from build123d import *

# Parameters (mm, degrees)
BOSS_EXTRUDE1_DEPTH     = 28.8
SKETCH3_R               = 3
SKETCH3_R_2             = 1.25
BOSS_EXTRUDE2_DEPTH     = 4
BOSS_EXTRUDE3_DEPTH     = 7.5
SKETCH5_W               = 15
SKETCH5_H               = 13.170644239
BOSS_EXTRUDE4_DEPTH     = 2
SKETCH6_R               = 0.725
BOSS_EXTRUDE5_DEPTH     = 1
CUT_EXTRUDE1_DEPTH      = 5
CUT_EXTRUDE1_DEPTH_BACK = 29.8
SKETCH8_W               = 6.2
SKETCH8_H               = 3.85
BOSS_EXTRUDE6_DEPTH     = 5
BOSS_EXTRUDE6_TAPER     = 10
FILLET1_R               = 0.5


with BuildPart() as part:
    # Sketch2 → Boss-Extrude1 (new body)
    with BuildSketch(Plane.XY):
        with BuildLine():
            Line((-7.5, 7), (7.5, 7))
            Line((7.5, 7), (7.5, -20.1))
            ThreePointArc((7.5, -20.1), (0, -27.6), (-7.5, -20.1))
            Line((-7.5, -20.1), (-7.5, 7))
        make_face()
    extrude(amount=-BOSS_EXTRUDE1_DEPTH)

    # Sketch3 → Boss-Extrude2 (add)
    with BuildSketch(Plane.XY):
        Circle(SKETCH3_R)
        Circle(SKETCH3_R_2, mode=Mode.SUBTRACT)
    extrude(amount=BOSS_EXTRUDE2_DEPTH)

    # Sketch4 → Boss-Extrude3 (add, symmetric)
    with BuildSketch(Plane(origin=(0, 0, 0), x_dir=(0, 0, -1), z_dir=(1, 0, 0))):
        Polygon((7.3, 7), (7.3, 13.6), (9.3, 13.6), (9.3, 7), (9.3, -35.1), (7.3, -35.1), align=None)
    extrude(amount=BOSS_EXTRUDE3_DEPTH, both=True)

    # Sketch5 → Boss-Extrude4 (add)
    with BuildSketch(Plane(origin=(0, 0, -9.3), x_dir=(-1, 0, 0), z_dir=(0, 0, -1))):
        with Locations((0, -21.914677881)):
            Rectangle(SKETCH5_W, SKETCH5_H)
    extrude(amount=BOSS_EXTRUDE4_DEPTH)

    # Sketch6 → Boss-Extrude5 (add)
    with BuildSketch(Plane(origin=(0, 0, -11.3), x_dir=(-1, 0, 0), z_dir=(0, 0, -1))):
        with Locations((-6.2, -27)):
            Circle(SKETCH6_R)
        with Locations((6.2, -27)):
            Circle(SKETCH6_R)
    extrude(amount=BOSS_EXTRUDE5_DEPTH)

    # Sketch7 → Cut-Extrude1 (cut, two sides)
    with BuildSketch(Plane.XY) as cut_extrude1_sk:
        with BuildLine():
            Line((-5, 12.036306817), (-5, 13.6))
            Line((-5, 13.6), (-2.7, 13.6))
            Line((-2.7, 13.6), (-2.7, 12.036306817))
            ThreePointArc((-2.7, 12.036306817), (-3.85, 8.4), (-5, 12.036306817))
        make_face()
        with BuildLine():
            Line((2.7, 13.6), (2.7, 12.036306817))
            ThreePointArc((2.7, 12.036306817), (3.85, 8.4), (5, 12.036306817))
            Line((5, 12.036306817), (5, 13.6))
            Line((5, 13.6), (2.7, 13.6))
        make_face()
        with BuildLine():
            Line((5, -33.536306817), (5, -35.1))
            Line((5, -35.1), (2.7, -35.1))
            Line((2.7, -35.1), (2.7, -33.536306817))
            ThreePointArc((2.7, -33.536306817), (3.85, -29.9), (5, -33.536306817))
        make_face()
        with BuildLine():
            Line((-2.7, -35.1), (-2.7, -33.536306817))
            ThreePointArc((-2.7, -33.536306817), (-3.85, -29.9), (-5, -33.536306817))
            Line((-5, -33.536306817), (-5, -35.1))
            Line((-5, -35.1), (-2.7, -35.1))
        make_face()
    extrude(amount=CUT_EXTRUDE1_DEPTH, mode=Mode.SUBTRACT)
    extrude(cut_extrude1_sk.sketch, amount=-CUT_EXTRUDE1_DEPTH_BACK, mode=Mode.SUBTRACT)

    # Sketch8 → Boss-Extrude6 (add)
    with BuildSketch(Plane(origin=(0, 7, 0), x_dir=(1, 0, 0), z_dir=(0, 1, 0))):
        with Locations((0, 24.875)):
            Rectangle(SKETCH8_W, SKETCH8_H)
    extrude(amount=BOSS_EXTRUDE6_DEPTH, taper=BOSS_EXTRUDE6_TAPER)

    # Fillet1
    fillet1_edges = [part.edges().sort_by_distance(p)[0] for p in [
        (-7.5, -6.55, -28.8),
        (0, -27.6, -28.8),
        (7.5, 7, -3.65),
        (-7.5, 7, -3.65),
        (7.5, -6.55, -28.8),
        (0, -27.6, 0),
        (-7.5, -6.55, 0),
        (0, 7, 0),
        (7.5, -6.55, 0),
        (0, 7, -28.8),
        (-7.5, 7, -19.05),
        (7.5, 7, -19.05),
    ]]
    fillet(fillet1_edges, radius=FILLET1_R)


solid = part.part
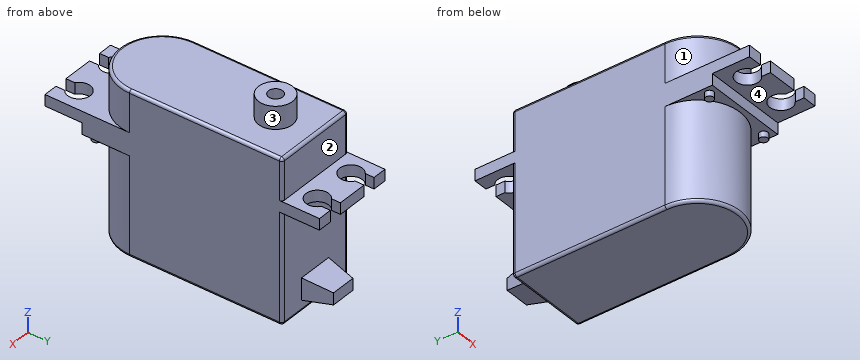
Could you check a few things on this model? Use its own coordinates, in mm. Face numbers are marked on the shaded views. A direction names the side the tool comes from. Round coordinates to 2 decimals unless told otherwise and drop trailing zeros. Write each loop counter-clockwise with the first axis right and the second up, starting at its lowest first coordinate (ties: lowest second). Pieces come first, ordered by that corner, then holes. Notation, with made-up numbers: (20.5, 34) - (75.5, 34) arc R13 ccw to (75.5, 54) - close; hole circle Ø1 at (-3, 76). An arc over 180 degrees is marked (long way). Use a Markdown table: item, result.
Q1. I want a section at D-D (z = -8.5). List the corners of the cut face in (x, y) for me.
Output values:
| item | result |
|---|---|
| outline | (-7.5, -35.1) - (-5, -35.1) - (-5, -33.54) arc R2 cw (long way) to (-2.7, -33.54) - (-2.7, -35.1) - (2.7, -35.1) - (2.7, -33.54) arc R2 cw (long way) to (5, -33.54) - (5, -35.1) - (7.5, -35.1) - (7.5, 13.6) - (5, 13.6) - (5, 12.04) arc R2 cw (long way) to (2.7, 12.04) - (2.7, 13.6) - (-2.7, 13.6) - (-2.7, 12.04) arc R2 cw (long way) to (-5, 12.04) - (-5, 13.6) - (-7.5, 13.6) - close |
Q2. Please list where these lines run through material, in increasing order: L1, parallel to X at y = 10.4, z = -7.95; L2, parallel to Z at x = 0.5, y = -18; L3, parallel to Y at x = 3.85, z = -8.75.
Output values:
| item | result |
|---|---|
| L1 | -7.5 to -5.85, -1.85 to 1.85, 5.85 to 7.5 |
| L2 | -28.8 to 0 |
| L3 | -29.9 to 8.4 |
Q3. For pin 1 (2 mm diameter, centred on x = 0.5, y = 0, fed in from +Z); pin 2 (2 mm diameter, centred on x = -2, y = -30.5, fed in from -Z); pin 3 (5 mm diameter, centred on x = 3.5, y = -14.5, fed in from +Z); pin 4 (0.7 mm diameter, centred on x = 6.5, y = -27, fed in from -Z), each with a flat end and sliding along its axis, tell me the tip position at first contact or that it passes through.
Output values:
| item | result |
|---|---|
| pin 1 | z = 4 |
| pin 2 | z = -9.3 |
| pin 3 | z = 0 |
| pin 4 | z = -12.3 |
Q4. I want a section at C-C (y = -14). List the corners of the cut face in (x, z) for me, plus the area to 3 significant figures.
Output values:
| item | result |
|---|---|
| outline | (-7.5, -28.3) arc R0.5 ccw to (-7, -28.8) - (7, -28.8) arc R0.5 ccw to (7.5, -28.3) - (7.5, -0.5) arc R0.5 ccw to (7, 0) - (-7, 0) arc R0.5 ccw to (-7.5, -0.5) - close |
| area | 432 mm2 |
Q5. I want a section at B-B (z = -13). List the corners of the cut face in (x, y) for me.
Output values:
| item | result |
|---|---|
| outline | (-7.5, -20.1) arc R7.5 ccw to (7.5, -20.1) - (7.5, 6.5) arc R0.5 ccw to (7, 7) - (-7, 7) arc R0.5 ccw to (-7.5, 6.5) - close |
Q6. I want a section at A-A (y = -31.9). List the corners of the cut face in (x, z) for me.
Output values:
| item | result |
|---|---|
| outline | (-7.5, -9.3) - (-5.85, -9.3) - (-5.85, -7.3) - (-7.5, -7.3) - close; (-1.85, -9.3) - (1.85, -9.3) - (1.85, -7.3) - (-1.85, -7.3) - close; (5.85, -9.3) - (7.5, -9.3) - (7.5, -7.3) - (5.85, -7.3) - close |
Q7. For the marked faces 1, 2, 3 and 4, which set-ups out of +Z, -Z, +X, -X, +Y, -Y let a thin tool reach every point of the face, with its end or its side?
Output values:
| item | result |
|---|---|
| face 1 | +Z, -Y |
| face 2 | +Z, +X, -X, +Y |
| face 3 | +Z |
| face 4 | -Z, +X, -X, -Y |
